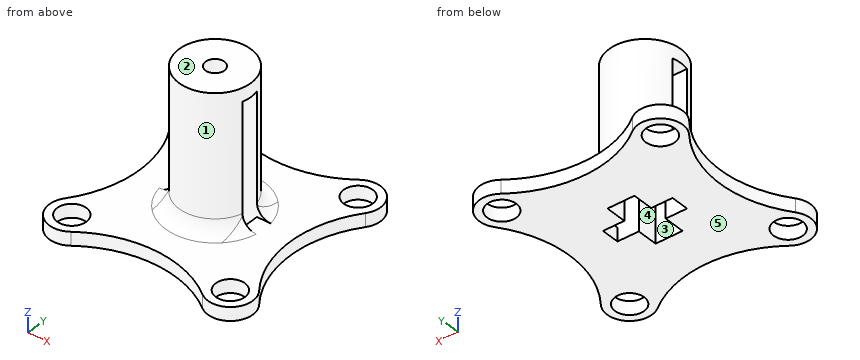
```python
from build123d import *

# Parameters (mm, degrees)
CROQUIS1_R              = 3.2499999999997446
CROQUIS1_R_2            = 3.249999999997429
CROQUIS1_R_3            = 3.249999999998684
SALIENTE_EXTRUIR1_DEPTH = 3
CORTAR_EXTRUIR2_REACH   = 34.211
SALIENTE_EXTRUIR2_DEPTH = 30
SALIENTE_EXTRUIR3_START = -3
CROQUIS4_R              = 8.000000000001583
CROQUIS4_R_2            = 2.1
SALIENTE_EXTRUIR3_DEPTH = 3
REDONDEO1_R             = 3


with BuildPart() as part:
    # Croquis1 → Saliente-Extruir1 (new body)
    with BuildSketch(Plane.XY):
        with BuildLine():
            ThreePointArc((-14.681197845286842, 21.680313336544412), (-21.21320343559782, 21.213203435599436), (-21.680313336542973, 14.681197845289143))
            ThreePointArc((-21.680313336542973, 14.681197845289143), (-16.79377171834698, -4.4873e-13), (-21.680313336546256, -14.681197845289011))
            ThreePointArc((-21.680313336546256, -14.681197845289011), (-21.213203435602523, -21.213203435600768), (-14.68119784529118, -21.680313336546952))
            ThreePointArc((-14.68119784529118, -21.680313336546952), (-1.37456e-12, -16.793771718350733), (14.681197845287352, -21.68031333655022))
            ThreePointArc((14.681197845287352, -21.68031333655022), (21.21320343559837, -21.213203435605198), (21.680313336544117, -14.68119784529431))
            ThreePointArc((21.680313336544117, -14.68119784529431), (16.79377171834798, -4.8379e-12), (21.680313336547112, 14.681197845283641))
            ThreePointArc((21.680313336547112, 14.681197845283641), (21.213203435602864, 21.21320343559648), (14.681197845291681, 21.680313336541143))
            ThreePointArc((14.681197845291681, 21.680313336541143), (1.87813e-12, 16.793771718344924), (-14.681197845286842, 21.680313336544412))
        make_face()
        with Locations((-17.677669529663632, 17.677669529664712)):
            Circle(CROQUIS1_R, mode=Mode.SUBTRACT)
        with Locations((17.67766952966688, 17.677669529661795)):
            Circle(CROQUIS1_R_2, mode=Mode.SUBTRACT)
        with Locations((17.67766952966414, -17.677669529670524)):
            Circle(CROQUIS1_R_3, mode=Mode.SUBTRACT)
        with Locations((-17.677669529667213, -17.677669529666943)):
            Circle(CROQUIS1_R, mode=Mode.SUBTRACT)
    extrude(amount=SALIENTE_EXTRUIR1_DEPTH)

    # Croquis2 → Cortar-Extruir2 (cut, up to next)
    with BuildSketch(Plane.XY.offset(3), mode=Mode.PRIVATE) as cortar_extruir2_sk1:
        Polygon((3.0000001045733526, -6.64999997299992), (3.000000062696712, -2.0000000028022047), (7.7459667027131305, -1.9999999600613383), (7.745966666690224, 2.00000009954332), (3.000000026673777, 2.000000056802398), (2.999999984797136, 6.650000027000114), (-3.0000001046098235, 6.649999972965725), (-3.000000062733182, 2.00000000276801), (-7.745966702749602, 1.9999999600271434), (-7.7459666821165225, -2.00000003997286), (-3.000000026710248, -1.9999999972319937), (-2.9999999848336065, -6.6500000270343085), align=None)
    cortar_extruir2_tool1 = extrude(cortar_extruir2_sk1.sketch, amount=-CORTAR_EXTRUIR2_REACH, mode=Mode.PRIVATE) & part.part
    add(cortar_extruir2_tool1.solids().sort_by_distance((0, 0, 3))[0], mode=Mode.SUBTRACT)

    # Croquis3 → Saliente-Extruir2 (add)
    with BuildSketch(Plane.XY.offset(3)):
        with BuildLine():
            Line((3.000000026673777, 2.000000056802398), (7.745966666690224, 2.00000009954332))
            ThreePointArc((7.7459666667244, 2.000000099552144), (-7.205040071e-08, 8.000000000013381), (-7.745966702749601, 1.9999999600271456))
            Line((-7.745966702749602, 1.9999999600271434), (-3.000000062733182, 2.00000000276801))
            Line((-3.000000062733182, 2.00000000276801), (-3.0000001046098235, 6.649999972965725))
            Line((-3.000000104609824, 6.649999972965725), (2.999999984797136, 6.650000027000114))
            Line((2.999999984797136, 6.650000027000113), (3.000000026673777, 2.000000056802398))
        make_face()
        with BuildLine():
            Line((3.000000062696712, -2.0000000028022047), (3.0000001045733526, -6.64999997299992))
            Line((3.0000001045733526, -6.64999997299992), (-2.9999999848336065, -6.6500000270343085))
            Line((-2.9999999848336065, -6.6500000270343085), (-3.000000026710248, -1.9999999972319937))
            Line((-3.0000000267102482, -1.9999999972319937), (-7.7459666821165225, -2.00000003997286))
            ThreePointArc((-7.745966682108257, -2.000000039970724), (4.126157047e-08, -8.000000000013381), (7.745966702739044, -1.9999999600680332))
            Line((7.7459667027131305, -1.9999999600613383), (3.000000062696712, -2.0000000028022047))
        make_face()
    extrude(amount=SALIENTE_EXTRUIR2_DEPTH)

    # Croquis4 → Saliente-Extruir3 (add)
    with BuildSketch(Plane.XY.offset(33).offset(SALIENTE_EXTRUIR3_START)):
        with Locations(Location((0, 0, 0), (0, 0, 165.52248811))):
            Circle(CROQUIS4_R)
        Circle(CROQUIS4_R_2, mode=Mode.SUBTRACT)
    extrude(amount=SALIENTE_EXTRUIR3_DEPTH)

    # Redondeo1
    # the kernel refuses this fillet: 3 mm, written as the material it adds along each edge
    with BuildSketch(Plane(origin=(4.4e-16, 4.4e-16, 3), x_dir=(-0.22595414891367588, 0.9741379381733866, 0), z_dir=(0.9741379381733866, 0.22595414891367588, 0))) as redondeo1_piece_1_section:
        with BuildLine():
            CenterArc((8.000000000013381 + REDONDEO1_R, REDONDEO1_R), REDONDEO1_R, 180, 90)
            Line((8.000000000013383, REDONDEO1_R), (8.000000000013381, 0))
            Line((8.000000000013381, 0), (8.000000000013381 + REDONDEO1_R, 0))
        make_face()
    redondeo1_piece_1 = revolve(axis=Axis((4.4e-16, 4.4e-16, 3), (0, 0, 1)), revolution_arc=333.88201682059855, mode=Mode.PRIVATE)
    redondeo1_piece_1 = split(redondeo1_piece_1, bisect_by=Plane(origin=(-7.745966692433063, -3.99557857e-08, 3), z_dir=(1.0, 5.158269811289524e-09, 0)), keep=Keep.TOP, mode=Mode.PRIVATE)
    redondeo1_piece_1 = split(redondeo1_piece_1, bisect_by=Plane(origin=(7.745966684701678, 6.975805769e-08, 3), z_dir=(-1.0, -9.005726474694729e-09, 0)), keep=Keep.TOP, mode=Mode.PRIVATE)
    add(redondeo1_piece_1)
    with BuildSketch(Plane(origin=(4.4e-16, 4.4e-16, 3), x_dir=(-0.22595414891367588, 0.9741379381733866, 0), z_dir=(0.9741379381733866, 0.22595414891367588, 0))) as redondeo1_piece_2_section:
        with BuildLine():
            CenterArc((8.000000000013381 + REDONDEO1_R, REDONDEO1_R), REDONDEO1_R, 180, 90)
            Line((8.000000000013383, REDONDEO1_R), (8.000000000013381, 0))
            Line((8.000000000013381, 0), (8.000000000013381 + REDONDEO1_R, 0))
        make_face()
    redondeo1_piece_2 = revolve(axis=Axis((4.4e-16, 4.4e-16, 3), (0, 0, 1)), revolution_arc=333.88201682059855, mode=Mode.PRIVATE)
    redondeo1_piece_2 = split(redondeo1_piece_2, bisect_by=Plane(origin=(-1.801144813e-08, 2.0000000297851828, 3), z_dir=(-9.005724153490957e-09, 1.0, 0)), keep=Keep.TOP, mode=Mode.PRIVATE)
    add(redondeo1_piece_2)
    with BuildSketch(Plane(origin=(4.4e-16, 4.4e-16, 3), x_dir=(-0.22595414891367588, 0.9741379381733866, 0), z_dir=(0.9741379381733866, 0.22595414891367588, 0))) as redondeo1_piece_3_section:
        with BuildLine():
            CenterArc((8.000000000013381 + REDONDEO1_R, REDONDEO1_R), REDONDEO1_R, 180, 90)
            Line((8.000000000013383, REDONDEO1_R), (8.000000000013381, 0))
            Line((8.000000000013381, 0), (8.000000000013381 + REDONDEO1_R, 0))
        make_face()
    redondeo1_piece_3 = revolve(axis=Axis((4.4e-16, 4.4e-16, 3), (0, 0, 1)), revolution_arc=333.88201682059855, mode=Mode.PRIVATE)
    redondeo1_piece_3 = split(redondeo1_piece_3, bisect_by=Plane(origin=(1.801144902e-08, -2.0000000298193776, 3), z_dir=(9.005724153490959e-09, -1.0, 0)), keep=Keep.TOP, mode=Mode.PRIVATE)
    add(redondeo1_piece_3)
    with BuildSketch(Plane(origin=(0, -4.4e-16, 3), x_dir=(0.22595415641693267, -0.9741379364329841, 0), z_dir=(-0.9741379364329841, -0.22595415641693267, 0))) as redondeo1_piece_4_section:
        with BuildLine():
            CenterArc((8.000000000013381 + REDONDEO1_R, REDONDEO1_R), REDONDEO1_R, 180, 90)
            Line((8.000000000013381, REDONDEO1_R), (8.000000000013381, 0))
            Line((8.000000000013381, 0), (8.000000000013381 + REDONDEO1_R, 0))
        make_face()
    redondeo1_piece_4 = revolve(axis=Axis((0, -4.4e-16, 3), (0, 0, 1)), revolution_arc=333.8820163789793, mode=Mode.PRIVATE)
    redondeo1_piece_4 = split(redondeo1_piece_4, bisect_by=Plane(origin=(-7.745966692433063, -3.995578659e-08, 3), z_dir=(1.0, 5.158269811289524e-09, 0)), keep=Keep.TOP, mode=Mode.PRIVATE)
    redondeo1_piece_4 = split(redondeo1_piece_4, bisect_by=Plane(origin=(7.745966684701678, 6.97580568e-08, 3), z_dir=(-1.0, -9.005726474694729e-09, 0)), keep=Keep.TOP, mode=Mode.PRIVATE)
    add(redondeo1_piece_4)
    with BuildSketch(Plane(origin=(0, -4.4e-16, 3), x_dir=(0.22595415641693267, -0.9741379364329841, 0), z_dir=(-0.9741379364329841, -0.22595415641693267, 0))) as redondeo1_piece_5_section:
        with BuildLine():
            CenterArc((8.000000000013381 + REDONDEO1_R, REDONDEO1_R), REDONDEO1_R, 180, 90)
            Line((8.000000000013381, REDONDEO1_R), (8.000000000013381, 0))
            Line((8.000000000013381, 0), (8.000000000013381 + REDONDEO1_R, 0))
        make_face()
    redondeo1_piece_5 = revolve(axis=Axis((0, -4.4e-16, 3), (0, 0, 1)), revolution_arc=333.8820163789793, mode=Mode.PRIVATE)
    redondeo1_piece_5 = split(redondeo1_piece_5, bisect_by=Plane(origin=(1.801144858e-08, -2.0000000298193776, 3), z_dir=(9.005724153490959e-09, -1.0, 0)), keep=Keep.TOP, mode=Mode.PRIVATE)
    add(redondeo1_piece_5)
    with BuildSketch(Plane(origin=(0, -4.4e-16, 3), x_dir=(0.22595415641693267, -0.9741379364329841, 0), z_dir=(-0.9741379364329841, -0.22595415641693267, 0))) as redondeo1_piece_6_section:
        with BuildLine():
            CenterArc((8.000000000013381 + REDONDEO1_R, REDONDEO1_R), REDONDEO1_R, 180, 90)
            Line((8.000000000013381, REDONDEO1_R), (8.000000000013381, 0))
            Line((8.000000000013381, 0), (8.000000000013381 + REDONDEO1_R, 0))
        make_face()
    redondeo1_piece_6 = revolve(axis=Axis((0, -4.4e-16, 3), (0, 0, 1)), revolution_arc=333.8820163789793, mode=Mode.PRIVATE)
    redondeo1_piece_6 = split(redondeo1_piece_6, bisect_by=Plane(origin=(-1.801144858e-08, 2.0000000297851828, 3), z_dir=(-9.005724153490957e-09, 1.0, 0)), keep=Keep.TOP, mode=Mode.PRIVATE)
    add(redondeo1_piece_6)


solid = part.part
```
Check sheet for the modelled part. Datum: model origin and axes. Units: mm. Face numbers are marked on the shaded views. A direction names the side the tool comes from. Round coordinates to 2 decimals unless told otherwise and drop trailing zeros. Order: outer loops, then holes, each group sorted by start corner. A loop starts at its lowest first (then second) coordinate and runs counter-clockwise, first axis right, second up. Notation, with made-up numbers: M 5,22 L 10,22 A33 ccw 10,61 Z; hole C 86,-30.75 d3. An arc over 180 degrees is marked long. Answer in a Markdown table with one row per item.
(1) Section check B-B on x = 0. Record the boundary of the cut face in (y, z), plus the area to 3 significant figures.
Findings:
| item | result |
|---|---|
| outline | M -16.79,0 L -6.65,0 L -6.65,30 L -2.1,30 L -2.1,33 L -8,33 L -8,6 A3 cw -11,3 L -16.79,3 Z; M 2.1,30 L 6.65,30 L 6.65,0 L 16.79,0 L 16.79,3 L 11,3 A3 cw 8,6 L 8,33 L 2.1,33 Z |
| area | 173 mm^2 |
(2) Draft check along X on the marked faces 1, 2 and 3. Enter one of: +X half, -X half, draft (parallel to the pull), parting line (faces both ways), or undercut.
Findings:
| item | result |
|---|---|
| face 1 | parting line |
| face 2 | draft |
| face 3 | undercut |
(3) Material ranges on line 1 along Z through (x, y) = (15, 12.5); line 2 along X through (y, z) = (-6.5, 21); line 3 along Y through (x, z) = (-1, 13), recorded low to high. Write a range as from..to.
Findings:
| item | result |
|---|---|
| line 1 | z = 0..3 |
| line 2 | x = -4.66..-3, 3..4.66 |
| line 3 | y = -7.94..-6.65, 6.65..7.94 |
(4) Set-up check for the marked faces 4 and 5: record each of +Z, -Z, +X, -X, +Y, -Y from which the full face is reachable in a straight line by a thin tool's end or side.
Findings:
| item | result |
|---|---|
| face 4 | -Z |
| face 5 | -Z, +X, -X, +Y, -Y |
(5) Section check C-C on y = 0. Record the boundary of the cut face in (x, z), plus the area to 3 significant figures.
Findings:
| item | result |
|---|---|
| outline | M -16.79,0 L -7.75,0 L -7.75,3 L -16.79,3 Z; M -8,30 L -2.1,30 L -2.1,33 L -8,33 Z; M 2.1,30 L 8,30 L 8,33 L 2.1,33 Z; M 7.75,0 L 16.79,0 L 16.79,3 L 7.75,3 Z |
| area | 89.7 mm^2 |
(6) Section check D-D on x = 19. Record the boundary of the cut face in (y, z).
Findings:
| item | result |
|---|---|
| outline | M -22.5,0 L -20.65,0 L -20.65,3 L -22.5,3 Z; M -14.71,0 L -10.16,0 L -10.16,3 L -14.71,3 Z; M 10.16,0 L 14.71,0 L 14.71,3 L 10.16,3 Z; M 20.65,0 L 22.5,0 L 22.5,3 L 20.65,3 Z |
(7) Section check A-A on z = 7. Record the boundary of the cut face in (x, y).
Findings:
| item | result |
|---|---|
| outline | M -7.75,-2 A8 ccw 7.75,-2 L 3,-2 L 3,-6.65 L -3,-6.65 L -3,-2 Z; M -7.75,2 L -3,2 L -3,6.65 L 3,6.65 L 3,2 L 7.75,2 A8 ccw Z |
(8) Gauge pin test, flat ends, axial feed: pin 1 (10 mm diameter, centred on x = -10.5, z = 27.5, fed in from -Y); pin 2 (4 mm diameter, centred on x = -8.5, z = 11.5, fed in from -Y); pin 3 (5 mm diameter, centred on x = -0.5, z = 16.5, fed in from +Y). Record the tip position at first contact, or that the pin passes through.
Findings:
| item | result |
|---|---|
| pin 1 | stops at y = -5.81 |
| pin 2 | stops at y = -4.66 |
| pin 3 | stops at y = 8 |
